For this review, take the finished solid that the model builds, in its own axes (mm). A direction names the side the tool comes from. Give positions to 0.01 mm unless a question says otherwise; leave off trailing zeros. Order: outer loops, then holes, each group sorted by start corner. A loop starts at its lowest first (then second) coordinate and runs counter-clockwise, first axis right, second up. Notation, with made-up numbers: (-23, 4.25) -> (-19, 4.25) arc R7 ccw to (-19, 10.25) -> close; hole circle Ø7 at (47, 70). An arc over 180 degrees is marked (long way). Return JSON: item names as keys, results as strings. Group by question number.
1) Add section A-A (x = 0). Give the boundary of the cut face in (y, z).
2) For faces 1 (the face through (1.894, 2.465, -5.369)), 2 (the face through (5.655, 2.465, 0.652)), 3 (the face through (-1.894, 2.465, 5.369)), 4 (the face through (-4.821, 2.465, 3.057)), list the 3-axis set-ups (+Z, -Z, +X, -X, +Y, -Y) from which the entire face can be reached by the end or side of a thin tool; tool diameter is ignored.
3) Insertion check: P1, Ø1, axis at x = -2, y = 2, coming from the -Z side; P2, Ø1.5, axis at y = 0.5, z = 4.5, coming from the +X side; P3, Ø3, axis at x = -3, y = 4, coming from the +Z side. Each pin has a flat end and moves straight along its axis. Give the tip position at first contact, or say it passes through.
4) The part is to be moulded in two halves that separate along X. For faces 5 (the face through (-5.396, 2.465, -1.863)), 6 (the face through (-0.62, 2.46, 5.67)), 7 (the face through (4.821, 2.465, -3.057)), 8 (the face through (3, 0, 1)), say which applies: released by +X, released by -X, zero draft, split by the parting line, or undercut.
5) Add section B-B (x = 2). Give the boundary of the cut face in (y, z), then the cut area to 3 significant figures.
6) To check wall thickness, follow line 1 along X through (y, z) = (1.25, 0); line 2 along X through (y, z) = (4.55, -3.75); line 3 along Z through (x, y) = (2, 3.8). State the ranges of each line that lie inside material, in increasing order.
from build123d import *

# Parameters (mm, degrees)
SKETCH1_R           = 3
BOSS_EXTRUDE1_DEPTH = 5


with BuildPart() as part:
    # Sketch1 → Boss-Extrude1 (new body)
    with BuildSketch(Plane(origin=(0, 0, 0), x_dir=(1, 0, 0), z_dir=(0, 1, 0))):
        with BuildLine():
            Line((-0.225, 6.145882768), (0, 6.145882768))
            Line((0, 6.145882768), (0.225, 6.145882768))
            ThreePointArc((0.225, 6.145882768), (0.619244207, 5.666854432), (0.7, 5.051732376))
            ThreePointArc((0.7, 5.051732376), (0.758505487, 4.796373711), (0.975, 4.648857386))
            Line((0.975, 4.648857386), (1.138618979, 4.611512422))
            ThreePointArc((1.138618979, 4.611512422), (1.39767873, 4.650486589), (1.561186325, 4.855172217))
            ThreePointArc((1.561186325, 4.855172217), (1.900836238, 5.374339414), (2.4638806, 5.634872881))
            Line((2.4638806, 5.634872881), (2.666598596, 5.53724904))
            Line((2.666598596, 5.53724904), (2.869316591, 5.439625199))
            ThreePointArc((2.869316591, 5.439625199), (3.016675742, 4.83697943), (2.82254274, 4.247734982))
            ThreePointArc((2.82254274, 4.247734982), (2.76445839, 3.992280195), (2.895508272, 3.765439131))
            Line((2.895508272, 3.765439131), (3.026720505, 3.660800866))
            ThreePointArc((3.026720505, 3.660800866), (3.277035533, 3.583513564), (3.513160551, 3.696985656))
            ThreePointArc((3.513160551, 3.696985656), (4.044432754, 4.017370563), (4.66475943, 4.007807313))
            Line((4.66475943, 4.007807313), (4.805044636, 3.831895229))
            Line((4.805044636, 3.831895229), (4.945329841, 3.655983146))
            ThreePointArc((4.945329841, 3.655983146), (4.816617649, 3.049081331), (4.386046274, 2.602421581))
            ThreePointArc((4.386046274, 2.602421581), (4.222876405, 2.397466625), (4.242525619, 2.136229475))
            Line((4.242525619, 2.136229475), (4.315342915, 1.985022802))
            ThreePointArc((4.315342915, 1.985022802), (4.507335258, 1.806781729), (4.769310245, 1.806565745))
            ThreePointArc((4.769310245, 1.806565745), (5.386979761, 1.864712202), (5.941725446, 1.586946354))
            Line((5.941725446, 1.586946354), (5.991792656, 1.367587574))
            Line((5.991792656, 1.367587574), (6.041859866, 1.148228793))
            ThreePointArc((6.041859866, 1.148228793), (5.662569359, 0.657275279), (5.080839552, 0.441666668))
            ThreePointArc((5.080839552, 0.441666668), (4.844901957, 0.327805387), (4.749258736, 0.083913373))
            Line((4.749258736, 0.083913373), (4.749258736, -0.083913373))
            ThreePointArc((4.749258736, -0.083913373), (4.844901957, -0.327805387), (5.080839552, -0.441666668))
            ThreePointArc((5.080839552, -0.441666668), (5.662569359, -0.657275279), (6.041859866, -1.148228793))
            Line((6.041859866, -1.148228793), (5.991792656, -1.367587574))
            Line((5.991792656, -1.367587574), (5.941725446, -1.586946354))
            ThreePointArc((5.941725446, -1.586946354), (5.386979761, -1.864712202), (4.769310245, -1.806565745))
            ThreePointArc((4.769310245, -1.806565745), (4.507335258, -1.806781729), (4.315342915, -1.985022802))
            Line((4.315342915, -1.985022802), (4.242525619, -2.136229475))
            ThreePointArc((4.242525619, -2.136229475), (4.222876405, -2.397466625), (4.386046274, -2.602421581))
            ThreePointArc((4.386046274, -2.602421581), (4.816617649, -3.049081331), (4.945329841, -3.655983146))
            Line((4.945329841, -3.655983146), (4.805044636, -3.831895229))
            Line((4.805044636, -3.831895229), (4.66475943, -4.007807313))
            ThreePointArc((4.66475943, -4.007807313), (4.044432754, -4.017370563), (3.513160551, -3.696985656))
            ThreePointArc((3.513160551, -3.696985656), (3.277035533, -3.583513564), (3.026720505, -3.660800866))
            Line((3.026720505, -3.660800866), (2.895508272, -3.765439131))
            ThreePointArc((2.895508272, -3.765439131), (2.76445839, -3.992280195), (2.82254274, -4.247734982))
            ThreePointArc((2.82254274, -4.247734982), (3.016675742, -4.83697943), (2.869316591, -5.439625199))
            Line((2.869316591, -5.439625199), (2.666598596, -5.53724904))
            Line((2.666598596, -5.53724904), (2.4638806, -5.634872881))
            ThreePointArc((2.4638806, -5.634872881), (1.900836238, -5.374339414), (1.561186325, -4.855172217))
            ThreePointArc((1.561186325, -4.855172217), (1.39767873, -4.650486589), (1.138618979, -4.611512422))
            Line((1.138618979, -4.611512422), (0.975, -4.648857386))
            ThreePointArc((0.975, -4.648857386), (0.758505487, -4.796373711), (0.7, -5.051732376))
            ThreePointArc((0.7, -5.051732376), (0.619244207, -5.666854432), (0.225, -6.145882768))
            Line((0.225, -6.145882768), (0, -6.145882768))
            Line((0, -6.145882768), (-0.225, -6.145882768))
            ThreePointArc((-0.225, -6.145882768), (-0.619244207, -5.666854432), (-0.7, -5.051732376))
            ThreePointArc((-0.7, -5.051732376), (-0.758505487, -4.796373711), (-0.975, -4.648857386))
            Line((-0.975, -4.648857386), (-1.138618979, -4.611512422))
            ThreePointArc((-1.138618979, -4.611512422), (-1.39767873, -4.650486589), (-1.561186325, -4.855172217))
            ThreePointArc((-1.561186325, -4.855172217), (-1.900836238, -5.374339414), (-2.4638806, -5.634872881))
            Line((-2.4638806, -5.634872881), (-2.666598596, -5.53724904))
            Line((-2.666598596, -5.53724904), (-2.869316591, -5.439625199))
            ThreePointArc((-2.869316591, -5.439625199), (-3.016675742, -4.83697943), (-2.82254274, -4.247734982))
            ThreePointArc((-2.82254274, -4.247734982), (-2.76445839, -3.992280195), (-2.895508272, -3.765439131))
            Line((-2.895508272, -3.765439131), (-3.026720505, -3.660800866))
            ThreePointArc((-3.026720505, -3.660800866), (-3.277035533, -3.583513564), (-3.513160551, -3.696985656))
            ThreePointArc((-3.513160551, -3.696985656), (-4.044432754, -4.017370563), (-4.66475943, -4.007807313))
            Line((-4.66475943, -4.007807313), (-4.805044636, -3.831895229))
            Line((-4.805044636, -3.831895229), (-4.945329841, -3.655983146))
            ThreePointArc((-4.945329841, -3.655983146), (-4.816617649, -3.049081331), (-4.386046274, -2.602421581))
            ThreePointArc((-4.386046274, -2.602421581), (-4.222876405, -2.397466625), (-4.242525619, -2.136229475))
            Line((-4.242525619, -2.136229475), (-4.315342915, -1.985022802))
            ThreePointArc((-4.315342915, -1.985022802), (-4.507335258, -1.806781729), (-4.769310245, -1.806565745))
            ThreePointArc((-4.769310245, -1.806565745), (-5.386979761, -1.864712202), (-5.941725446, -1.586946354))
            Line((-5.941725446, -1.586946354), (-5.991792656, -1.367587574))
            Line((-5.991792656, -1.367587574), (-6.041859866, -1.148228793))
            ThreePointArc((-6.041859866, -1.148228793), (-5.662569359, -0.657275279), (-5.080839552, -0.441666668))
            ThreePointArc((-5.080839552, -0.441666668), (-4.844901957, -0.327805387), (-4.749258736, -0.083913373))
            Line((-4.749258736, -0.083913373), (-4.749258736, 0.083913373))
            ThreePointArc((-4.749258736, 0.083913373), (-4.844901957, 0.327805387), (-5.080839552, 0.441666668))
            ThreePointArc((-5.080839552, 0.441666668), (-5.662569359, 0.657275279), (-6.041859866, 1.148228793))
            Line((-6.041859866, 1.148228793), (-5.991792656, 1.367587574))
            Line((-5.991792656, 1.367587574), (-5.941725446, 1.586946354))
            ThreePointArc((-5.941725446, 1.586946354), (-5.386979761, 1.864712202), (-4.769310245, 1.806565745))
            ThreePointArc((-4.769310245, 1.806565745), (-4.507335258, 1.806781729), (-4.315342915, 1.985022802))
            Line((-4.315342915, 1.985022802), (-4.242525619, 2.136229475))
            ThreePointArc((-4.242525619, 2.136229475), (-4.222876405, 2.397466625), (-4.386046274, 2.602421581))
            ThreePointArc((-4.386046274, 2.602421581), (-4.816617649, 3.049081331), (-4.945329841, 3.655983146))
            Line((-4.945329841, 3.655983146), (-4.805044636, 3.831895229))
            Line((-4.805044636, 3.831895229), (-4.66475943, 4.007807313))
            ThreePointArc((-4.66475943, 4.007807313), (-4.044432754, 4.017370563), (-3.513160551, 3.696985656))
            ThreePointArc((-3.513160551, 3.696985656), (-3.277035533, 3.583513564), (-3.026720505, 3.660800866))
            Line((-3.026720505, 3.660800866), (-2.895508272, 3.765439131))
            ThreePointArc((-2.895508272, 3.765439131), (-2.76445839, 3.992280195), (-2.82254274, 4.247734982))
            ThreePointArc((-2.82254274, 4.247734982), (-3.016675742, 4.83697943), (-2.869316591, 5.439625199))
            Line((-2.869316591, 5.439625199), (-2.666598596, 5.53724904))
            Line((-2.666598596, 5.53724904), (-2.4638806, 5.634872881))
            ThreePointArc((-2.4638806, 5.634872881), (-1.900836238, 5.374339414), (-1.561186325, 4.855172217))
            ThreePointArc((-1.561186325, 4.855172217), (-1.39767873, 4.650486589), (-1.138618979, 4.611512422))
            Line((-1.138618979, 4.611512422), (-0.975, 4.648857386))
            ThreePointArc((-0.975, 4.648857386), (-0.758505487, 4.796373711), (-0.7, 5.051732376))
            ThreePointArc((-0.7, 5.051732376), (-0.619244207, 5.666854432), (-0.225, 6.145882768))
        make_face()
        with Locations(Location((0, 0, 0), (0, 0, 270))):
            Circle(SKETCH1_R, mode=Mode.SUBTRACT)
    extrude(amount=BOSS_EXTRUDE1_DEPTH)


solid = part.part
Evaluation:
{
 "1": {"outline": "(0, -6.15) -> (5, -6.15) -> (5, -3) -> (0, -3) -> close; (0, 3) -> (5, 3) -> (5, 6.15) -> (0, 6.15) -> close"},
 "2": {"face 1": "-Z, +Y, -Y", "face 2": "+X, +Y, -Y", "face 3": "+Z, +Y, -Y", "face 4": "-X, +Y, -Y"},
 "3": {"P1": "z = -5.63", "P2": "x = 4.87", "P3": "z = 5.63"},
 "4": {"face 5": "undercut", "face 6": "undercut", "face 7": "released by +X", "face 8": "zero draft"},
 "5": {"outline": "(0, -5.45) -> (5, -5.45) -> (5, -2.24) -> (0, -2.24) -> close; (0, 2.24) -> (5, 2.24) -> (5, 5.45) -> (0, 5.45) -> close", "area": "32.1 mm^2"},
 "6": {"line 1": "-4.75 to -3, 3 to 4.75", "line 2": "-4.87 to -3.57, -2.91 to 2.91, 3.57 to 4.87", "line 3": "-5.45 to -2.24, 2.24 to 5.45"}
}
